Could you check a few things on this drawing? It's one solid part, dimensions in mm from its lowest x, y, z. Give positions to 0.01 mm unless a question says otherwise; leave off trailing zeros. Order: outer loops, then holes, each group sorted by start corner. A loop starts at its lowest first (then second) coordinate and runs counter-clockwise, first axis right, second up.
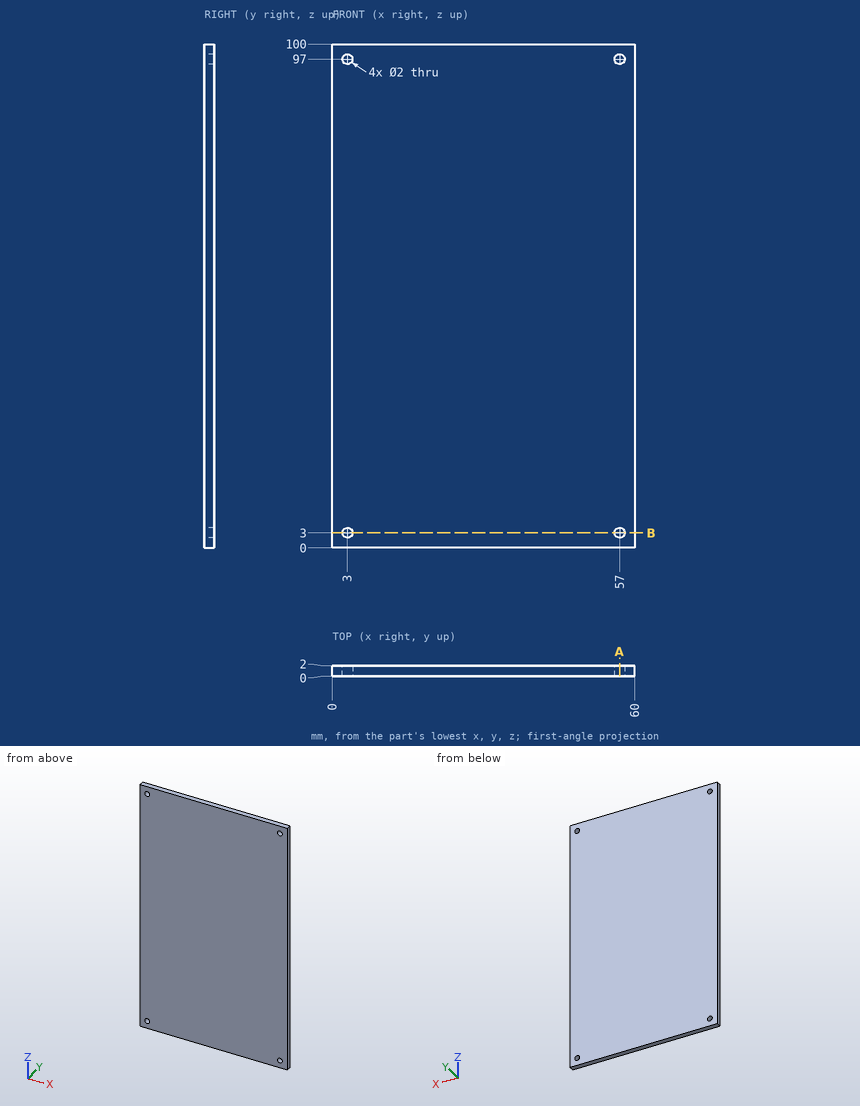
Q1. If we section it at B-B on z = 3: List the corners of the cut face in (x, y) for me, plus the area to 3 significant figures.
Filled sheet:
outline: (0, 0) - (2, 0) - (2, 2) - (0, 2) - close; (4, 0) - (56, 0) - (56, 2) - (4, 2) - close; (58, 0) - (60, 0) - (60, 2) - (58, 2) - close
area: 112 mm2
Q2. I need wall thicknesses on L1, parallel to X at y = 0.8, z = 97; L2, parallel to Z at x = 57, y = 0.8. Which ranges of each line are inside material? Lowest first, please.
Filled sheet:
L1: x = 0 to 2, 4 to 56, 58 to 60
L2: z = 0 to 2, 4 to 96, 98 to 100
Q3. I'm going to push a flat-ended pin straight in: P1, Ø1.2, axis at x = 57, z = 97, coming from the +Y side. Where does the tip first touch, or does it pass through?
Filled sheet:
P1: passes through
Q4. If we section it at A-A on x = 57: List the corners of the cut face in (y, z) for me, plus the area to 3 significant figures.
Filled sheet:
outline: (0, 0) - (2, 0) - (2, 2) - (0, 2) - close; (0, 4) - (2, 4) - (2, 96) - (0, 96) - close; (0, 98) - (2, 98) - (2, 100) - (0, 100) - close
area: 192 mm2
